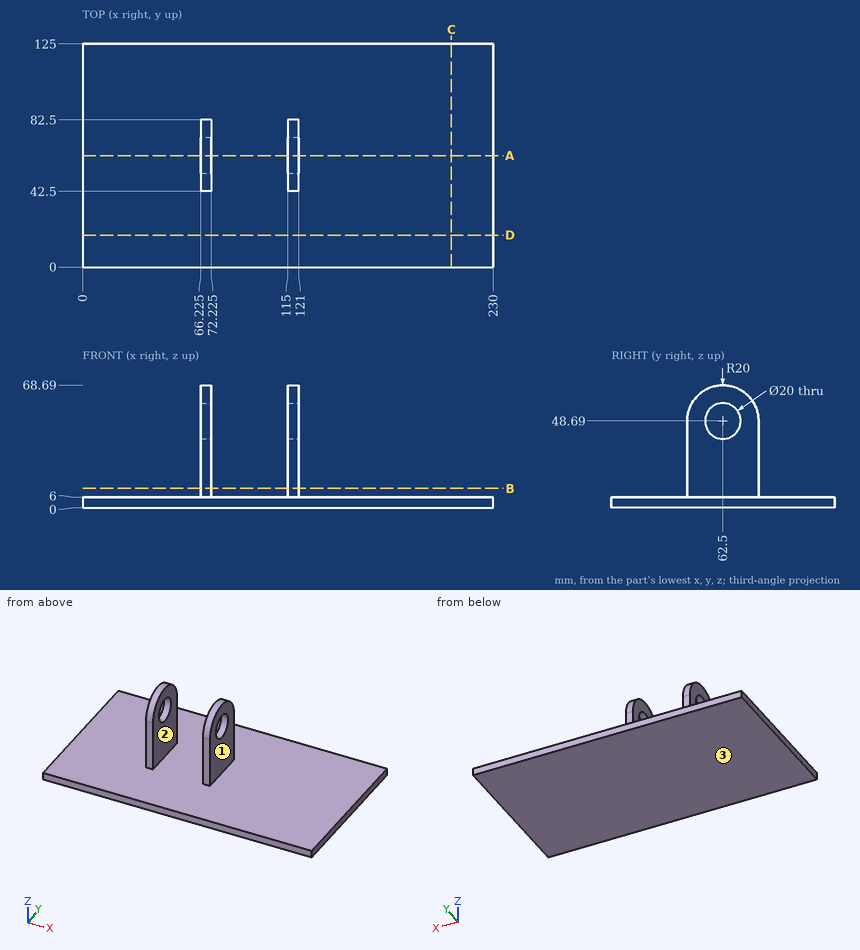
Job drawing, mm, ordinate dimensions from the low corner. One solid piece. A direction names the side the tool comes from. Give positions to 0.01 mm unless a question says otherwise; leave off trailing zeros. Loops run counter-clockwise (first coordinate to the right, second up) from the corner with the lowest first, then second, coordinate; pieces in that order, holes last. Notation, with made-up numbers: M 0,-16.5 L 33,-16.5 A29 ccw 33,7.5 Z; hole C 71.5,50.25 d3. An arc over 180 degrees is marked long. Return JSON: item names as keys, results as strings.
1) Drill centre lines: line 1 (Z direction, x = 119.8, y = 62.5); line 2 (X direction, y = 63.5, z = 10) (1 decimal); line 3 (Z direction, x = 91, y = 62). Where is each one in solid material? Low to high.
Calculated:
{"line 1": "z = 0 to 38.69, 58.69 to 68.69", "line 2": "x = 66.2 to 72.2, 115 to 121", "line 3": "z = 0 to 6"}
2) Saw through at D-D, the plane y = 18. List the corners of the cut face in (x, z).
Calculated:
{"outline": "M 0,0 L 230,0 L 230,6 L 0,6 Z"}
3) Flat gauge pins, fed straight in: pin 1 Ø8 at (y, z) = (92.5, 10.5) entering from -X; pin 2 Ø8 at (x, y) = (172, 81.5) entering from +Z; pin 3 Ø1.8 at (x, z) = (68.5, 36) entering from +Y; pin 4 Ø1.8 at (x, z) = (117, 26) entering from -Y. Where does each tip first touch, or does it go through?
Calculated:
{"pin 1": "passes through", "pin 2": "stops at z = 6", "pin 3": "stops at y = 82.5", "pin 4": "stops at y = 42.5"}
4) 3-axis set-ups, long thin cutter, end or side, ignore diameter. For the marked faces 1, 2 and 3: which of +Z, -Z, +X, -X, +Y, -Y reach the whole face in a straight line?
Calculated:
{"face 1": "+Z, +X, +Y, -Y", "face 2": "+Z, +Y, -Y", "face 3": "-Z, +X, -X, +Y, -Y"}
5) Saw through at B-B, the plane z = 11. List the corners of the cut face in (x, y) (1 decimal).
Calculated:
{"outline": "M 66.2,42.5 L 72.2,42.5 L 72.2,82.5 L 66.2,82.5 Z; M 115,42.5 L 121,42.5 L 121,82.5 L 115,82.5 Z"}
6) Saw through at A-A, the plane y = 62.5. List the corners of the cut face in (x, z) (1 decimal).
Calculated:
{"outline": "M 0,0 L 230,0 L 230,6 L 121,6 L 121,38.7 L 115,38.7 L 115,6 L 72.2,6 L 72.2,38.7 L 66.2,38.7 L 66.2,6 L 0,6 Z; M 66.2,58.7 L 72.2,58.7 L 72.2,68.7 L 66.2,68.7 Z; M 115,58.7 L 121,58.7 L 121,68.7 L 115,68.7 Z"}
7) Saw through at C-C, the plane x = 206.5. List the corners of the cut face in (y, z), then the cut area to 3 significant figures.
Calculated:
{"outline": "M 0,0 L 125,0 L 125,6 L 0,6 Z", "area": "750 mm2"}
